```python
from build123d import *

# Parameters (mm, degrees)
F1_DEPTH = 12
F2_R     = 3.1
F3_DEPTH = 12.001
F4_R     = 1.75
F5_DEPTH = 6.001
F6_R     = 3.25
F7_DEPTH = 3
F8_W     = 2.8
F8_H     = 4
F9_DEPTH = 13.90725


with BuildPart() as f1:
    # F0 (on Top) → F1 (new body)
    with BuildSketch(Plane.XY):
        Polygon((-13.285446, 0), (19.808304, 0), (19.808304, 6), (-27.191696, 6), (-27.191696, -5), (-13.285446, -5), align=None)
    extrude(amount=F1_DEPTH)

    # F2 (on face) → F3 (cut, through all)
    with BuildSketch(Plane.XY.offset(12)):
        with Locations((-20.238571, -5)):
            Circle(F2_R)
    extrude(amount=-F3_DEPTH, mode=Mode.SUBTRACT)

    # F4 (on face) → F5 (cut, through all)
    with BuildSketch(Plane.XZ):
        with Locations((13.808304, 6)):
            Circle(F4_R)
        with Locations((-4.391696, 6)):
            Circle(F4_R)
    extrude(amount=-F5_DEPTH, mode=Mode.SUBTRACT)

    # F6 (on face) → F7 (cut)
    with BuildSketch(Plane.XZ):
        with Locations((-4.391696, 6)):
            Circle(F6_R)
        with Locations((13.808304, 6)):
            Circle(F6_R)
    extrude(amount=-F7_DEPTH, mode=Mode.SUBTRACT)

    # F8 (on face) → F9 (cut, through all)
    with BuildSketch(Plane.YZ.offset(-13.285446)):
        with Locations((-1.4, 5.94657)):
            Rectangle(F8_W, F8_H)
    extrude(amount=-F9_DEPTH, mode=Mode.SUBTRACT)


solid = f1.part
```
Geometry check sheet. Reference: the model listing, model coordinates, mm. A direction names the side the tool comes from. Give positions to 0.01 mm unless a question says otherwise; leave off trailing zeros. Write each loop counter-clockwise with the first axis right and the second up, starting at its lowest first coordinate (ties: lowest second). Pieces come first, ordered by that corner, then holes.
1) Section check A-A, the plane z = 6. Record the boundary of the cut face in (x, y), and give its area (3 significant figures).
2) Release check for a two-part mould opening along X. For faces 1 (the flat face through (-27.192, 1, 6)), 2 (the cylindrical face through (16.9, 1.5, 7)), 3 (the flat face through (-15, -5, 6)), 4 (the flat face through (-13.285, -3, 6)) record: pulls with the +X half, pulls with the -X half, needs draft (parallel to the pull), parting line crosses it, or undercut.
3) Section check B-B, the plane x = -4.5. Record the boundary of the cut face in (y, z), and give its area (3 significant figures).
4) Gauge pin test, flat ends, axial feed: pin 1 (1 mm diameter, centred on x = 13, y = -1.5, fed in from +Z); pin 2 (4 mm diameter, centred on x = 13.81, z = 6, fed in from -Y); pin 3 (5 mm diameter, centred on x = -5.5, z = 4.5, fed in from -Y); pin 4 (5.5 mm diameter, centred on y = -3.5, z = 7.5, fed in from +X). Record the tip position at first contact, or that the pin passes through.
5) Section check D-D, the plane z = 8.75. Record the boundary of the cut face in (x, y).
6) Access from +Z, -Z, +X, -X, +Y, -Y to the whole of each face (thin tool, end or side, straight path). Record for faces 5 (the flat face through (15.2, 3, 4.6)), 6 (the flat face through (-16, -2.8, 6)), 7 (the flat face through (-3, 6, 3)).
7) Section check C-C, the plane z = 1. Record the boundary of the cut face in (x, y), and give its area (3 significant figures).
8) Material ranges on L1, parallel to Z at x = -14, y = -1; L2, parallel to X at y = 2.5, z = 6.75; L3, parallel to Y at x = -13, z = 3, recorded low to high.
Computed:
1. outline: (-27.19, -5) - (-23.34, -5) arc R3.1 cw to (-22.42, -2.8) - (-27.19, -2.8) - close; (-27.19, 0) - (-7.64, 0) - (-7.64, 3) - (-6.14, 3) - (-6.14, 6) - (-27.19, 6) - close; (-18.05, -2.8) arc R3.1 cw to (-17.14, -5) - (-13.29, -5) - (-13.29, -2.8) - close; (-2.64, 3) - (-1.14, 3) - (-1.14, 0) - (10.56, 0) - (10.56, 3) - (12.06, 3) - (12.06, 6) - (-2.64, 6) - close; (15.56, 3) - (17.06, 3) - (17.06, 0) - (19.81, 0) - (19.81, 6) - (15.56, 6) - close
1. area: 240 mm2
2. face 1: pulls with the -X half
2. face 2: undercut
2. face 3: needs draft
2. face 4: pulls with the +X half
3. outline: (0, 0) - (6, 0) - (6, 4.25) - (3, 4.25) - (3, 2.75) - (0, 2.75) - close; (0, 9.25) - (3, 9.25) - (3, 7.75) - (6, 7.75) - (6, 12) - (0, 12) - close
3. area: 42.0 mm2
4. pin 1: passes through
4. pin 2: stops at y = 3
4. pin 3: stops at y = 0
4. pin 4: stops at x = -13.29
5. outline: (-27.19, -5) - (-23.34, -5) arc R3.1 cw to (-17.14, -5) - (-13.29, -5) - (-13.29, 0) - (-6.12, 0) - (-6.12, 3) - (-2.66, 3) - (-2.66, 0) - (12.08, 0) - (12.08, 3) - (15.54, 3) - (15.54, 0) - (19.81, 0) - (19.81, 6) - (-27.19, 6) - close
6. face 5: -Y
6. face 6: +X, -X
6. face 7: +Z, -Z, +X, -X, +Y
7. outline: (-27.19, -5) - (-23.34, -5) arc R3.1 cw to (-17.14, -5) - (-13.29, -5) - (-13.29, 0) - (19.81, 0) - (19.81, 6) - (-27.19, 6) - close
7. area: 336 mm2
8. L1: z = 0 to 3.95, 7.95 to 12
8. L2: x = -27.19 to -7.55, -1.23 to 10.65, 16.97 to 19.81
8. L3: y = 0 to 6
